Work out the finished part from the listing and answer in its coordinate system (mm). Coordinates: 2 decimals unless noted, no trailing zeros. Write each loop counter-clockwise with the first axis right and the second up, starting at its lowest first coordinate (ties: lowest second). Pieces come first, ordered by that corner, then holes. Notation, with made-up numbers: M -31.75,89 L 13.25,89 A12 cw 13.25,94 Z; hole C 60,-35 d2. An arc over 180 degrees is marked long. Answer as CSV lines item,"result". Start each with the question number.
(1) A cutting plane is placed at B-B on y = -12.5. Give the vertices of the cut face in (x, z).
(2) A flat-ended cylindrical pin translates along its axis: P1, Ø5, axis at y = -2, z = -1.5, coming from the -X side. Find the tip coordinate at first contact, or state that the pin passes through.
(3) The mould has two halves that part along Z. Classify faces 1 (the flat face through (10, 0, 1)), 2 (the cylindrical face through (4.937, -15.879, 33.685)), 3 (the flat face through (4, 0, -50)): released by +Z, released by -Z, zero draft, split by the parting line, or undercut.
(4) Find the intervals of material crossed by L1, parallel to Y at x = 3, z = 30; L2, parallel to Z at x = 6, y = -12.5; L3, parallel to Z at x = 2.75, y = -16.5, in increasing order. Write a range as [from, to].
(5) A cutting plane is placed at C-C on x = 4. Give the vertices of the cut face in (y, z), then the cut area to 3 significant figures.
(6) A cutting plane is placed at A-A on z = 30. Give the vertices of the cut face in (x, y), then the cut area to 3 significant figures.
Autodesk Inventor part; units mm, degrees
ref_plane "YZ Plane" through (0, 0, 0) normal (1, 0, 0) x (0, 1, 0)
ref_plane "XZ Plane" through (0, 0, 0) normal (0, 1, 0) x (-1, 0, 0)
ref_plane "XY Plane" through (0, 0, 0) normal (0, 0, 1) x (1, 0, 0)
sketch "草圖1" plane through (0, 0, 0) normal (1, 0, 0) x (0, 1, 0)
  line L0 (-35, 0) -> (35, 0)
  line L1 (0, -70) -> (0, 70)
  line L2 (-25, 50) -> (25, 50)
  line L3 (25, 50) -> (25, -50)
  line L4 (25, -50) -> (-25, -50)
  line L5 (-25, -50) -> (-25, 50)
  line L6 (-25, 50) -> (25, -50) construction
  line L7 (25, 50) -> (-25, -50) construction
  point P0 (0, 0)
  dimension "d0" = 50
  dimension "d1" = 100
extrude "擠出1" add sketch "草圖1" along normal blind 10
fillet "圓角1" radius 1 4 edges at (5, 25, 50) (5, -25, 50) (5, -25, -50) (5, 25, -50)
chamfer "倒角1" distance 1 angle 45 8 edges at (10, 0, 50) (10, -24.7071, 49.7071) (10, -25, 0) (10, -24.7071, -49.7071) (10, 0, -50) (10, 24.7071, -49.7071) (10, 25, 0) (10, 24.7071, 49.7071)
sketch "草圖2" plane through (10, 0, 0) normal (1, 0, 0) x (0, 0, -1)
  line L0 (-50, 24) -> (-50, -24)
  line L1 (-30, 24) -> (-30, -24)
  line L2 (0, -35) -> (0, 35)
  line L3 (70, 0) -> (-70, 0)
  line L4 (70, 12.5) -> (-70, 12.5)
  line L5 (70, -12.5) -> (-70, -12.5)
  point P0 (0, 0)
  point P1 (-30, 12.5)
  point P2 (-30, -12.5)
  dimension "d8" = 20
  dimension "d9" = 12.5
  dimension "d10" = 12.5
hole "孔1" at (10, 12.5, 30) at (10, -12.5, 30) direction (-1, 0, 0) diameter 10 end through all
thread "螺紋1"
thread "螺紋2"
chamfer "倒角2" distance 0.5 angle 45 4 edges at (10, -12.5, 35) (10, 12.5, 35) (0, -12.5, 35) (0, 12.5, 35)
properties part number "exercise3-4"
Here are the results:
1,outline,"M 0,-50 L 9,-50 L 10,-49 L 10,24.5 L 9.5,25 L 0.5,25 L 0,24.5 Z; M 0,35.5 L 0.5,35 L 9.5,35 L 10,35.5 L 10,49 L 9,50 L 0,50 Z"
2,P1,"stops at x = 0"
3,face 1,"zero draft"
3,face 2,"undercut"
3,face 3,"released by -Z"
4,L1,"y = [-25, -17.5], [-7.5, 7.5], [17.5, 25]"
4,L2,"z = [-50, 25], [35, 50]"
4,L3,"z = [-50, 27], [33, 50]"
5,outline,"M -25,-49 A1 ccw -24,-50 L 24,-50 A1 ccw 25,-49 L 25,49 A1 ccw 24,50 L -24,50 A1 ccw -25,49 Z; hole C -12.5,30 d10; hole C 12.5,30 d10"
5,area,"4,840 mm^2"
6,outline,"M 0,-25 L 9,-25 L 10,-24 L 10,-18 L 9.5,-17.5 L 0.5,-17.5 L 0,-18 Z; M 0,-7 L 0.5,-7.5 L 9.5,-7.5 L 10,-7 L 10,7 L 9.5,7.5 L 0.5,7.5 L 0,7 Z; M 0,18 L 0.5,17.5 L 9.5,17.5 L 10,18 L 10,24 L 9,25 L 0,25 Z"
6,area,"298 mm^2"
